from build123d import *

# Parameters (mm, degrees)
F1_DEPTH = 2
F0_W     = 5
F0_H     = 5
F2_DEPTH = 5
F3_R     = 1
F4_DEPTH = 5
F5_R     = 2


with BuildPart() as f1:
    # F0 (on Front) → F1 (new body)
    with BuildSketch(Plane.XZ):
        Polygon((122.376468, -10.288223), (122.376468, 18.867619), (-122.376468, 47.667619), (-122.376468, 27.667619), (-122.376468, 22.667619), (-122.376468, -47.667619), (122.376468, -18.867619), (122.376468, -15.288223), (117.376468, -15.288223), (117.376468, -10.288223), align=None)
    extrude(amount=F1_DEPTH)

    # F0 (on Front) → F2 (join)
    with BuildSketch(Plane.XZ):
        with Locations((119.876468, -12.788223)):
            Rectangle(F0_W, F0_H)
    extrude(amount=F2_DEPTH)

    # F3 (on face) → F4 (join)
    with BuildSketch(Plane.XY.offset(-10.288223)):
        with Locations((119.876468, -3.5)):
            Circle(F3_R)
    extrude(amount=F4_DEPTH)

    # F5
    f5_edges = [f1.edges().sort_by_distance(p)[0] for p in [
        (119.876468, -5, -15.288223),
        (122.376468, -5, -12.788223),
        (122.376468, -3.5, -15.288223),
        (117.376468, -3.5, -15.288223),
        (117.376468, -5, -12.788223),
    ]]
    fillet(f5_edges, radius=F5_R)


solid = f1.part
Verification items for the finished model (mm, model axes). Give positions to 0.01 mm unless a question says otherwise; leave off trailing zeros. Write each loop counter-clockwise with the first axis right and the second up, starting at its lowest first coordinate (ties: lowest second). Pieces come first, ordered by that corner, then holes. Notation, with made-up numbers: M -23,88.5 L 4,88.5 A10 ccw 4,101.5 Z; hole C 78,53 d9. An arc over 180 degrees is marked long. Write item = value, one per line.
(1) Sectioned sample at A-A (z = 10). Record the cut outline in (x, y).
Found:
outline = M -122.38,-2 L 122.38,-2 L 122.38,0 L -122.38,0 Z
(2) Material ranges on line 1 (Y direction, x = -34.5, z = 8.5); line 2 (Z direction, x = -87, y = -1.15); line 3 (X direction, y = -2.7, z = -11.5), recorded low to high.
Found:
line_1 = -2 to 0
line_2 = -43.5 to 43.5
line_3 = 117.38 to 122.38
(3) Sectioned sample at B-B (x = 36). Record the cut outline in (y, z).
Found:
outline = M -2,-29.03 L 0,-29.03 L 0,29.03 L -2,29.03 Z
(4) Go/stop test with flat-tipped pins: pin 1 Ø3 at (y, z) = (-3, 35.5) entering from -X; pin 2 Ø1 at (x, y) = (-68, -2) entering from +Z; pin 3 Ø0.8 at (x, y) = (120, -2.5) entering from -Z; pin 4 Ø0.9 at (x, y) = (120, -3) entering from +Z. Record where each tip stops, or that it passes through.
Found:
pin_1 = -122.38
pin_2 = 41.33
pin_3 = -15.29
pin_4 = -5.29
